```python
from build123d import *

# Parameters (mm, degrees)
F0_W     = 83.5
F0_H     = 70.2625
F0_W_2   = 8
F0_H_2   = 3.175
F0_W_3   = 77.5
F0_H_3   = 24
F0_R     = 1
F0_W_4   = 6
F0_W_5   = 17
F0_H_4   = 31
F0_W_6   = 10
F0_H_5   = 10
F0_R_2   = 1.2
F1_DEPTH = 3.175


# Not quite as in the source:
# - a length typed as a fraction of an inch, garbled in the dataset ("3 / 203.2 mm" for 3/8 in), is restored
# - a feature names something its author has since deleted; it is built from what else it names


with BuildPart() as f1:
    # F0 (on Top) → F1 (new body)
    with BuildSketch(Plane.XY):
        with Locations((2.5199788651, 27.2772044539)):
            Rectangle(F0_W, F0_H)
        with Locations((-12.4800211349, -3.1790455461)):
            Rectangle(F0_W_2, F0_H_2, mode=Mode.SUBTRACT)
        with BuildLine():
            ThreePointArc((-0.9800211349, -4.6790455461), (-2.0406813067, -2.1183853743), (0.5199788651, -3.1790455461))
            ThreePointArc((0.5199788651, -3.1790455461), (0.0806390368, -4.2397057179), (-0.9800211349, -4.6790455461))
        make_face(mode=Mode.SUBTRACT)
        with Locations((10.5199788651, -3.1790455461)):
            Rectangle(F0_W_2, F0_H_2, mode=Mode.SUBTRACT)
        with Locations((2.5199788651, 13.4084544539)):
            Rectangle(F0_W_3, F0_H_3, mode=Mode.SUBTRACT)
        Polygon((-36.2300211349, 34.4084544539), (-36.230021135, 44.4084544539), (-36.230021135, 54.4084544539), (-26.230021135, 54.4084544539), (-26.230021135, 44.4084544539), (-26.2300211349, 34.4084544539), align=None, mode=Mode.SUBTRACT)
        with Locations((-14.980021135, 29.4084544539)):
            Circle(F0_R, mode=Mode.SUBTRACT)
        Polygon((-21.230021135, 31.9084544539), (-21.230021135, 55.9084544539), (-8.730021135, 55.9084544539), (-8.730021135, 43.9084544539), (-8.730021135, 31.9084544539), align=None, mode=Mode.SUBTRACT)
        with Locations((-14.980021135, 58.4084544539)):
            Circle(F0_R, mode=Mode.SUBTRACT)
        with Locations((21.2699788651, 35.3209544539)):
            Rectangle(F0_W_4, F0_H_2, mode=Mode.SUBTRACT)
        with Locations((2.7699788651, 43.9084544539)):
            Rectangle(F0_W_5, F0_H_4, mode=Mode.SUBTRACT)
        with BuildLine():
            ThreePointArc((29.7699788651, 33.8209544539), (28.7093186933, 36.3816146257), (31.2699788651, 35.3209544539))
            ThreePointArc((31.2699788651, 35.3209544539), (30.8306390368, 34.2602942821), (29.7699788651, 33.8209544539))
        make_face(mode=Mode.SUBTRACT)
        with Locations((38.2699788651, 35.3209544539)):
            Rectangle(F0_W_4, F0_H_2, mode=Mode.SUBTRACT)
        Polygon((14.2699788651, 54.4084544539), (24.2699788651, 54.4084544539), (34.2699788651, 54.4084544539), (34.2699788651, 44.4084544539), (24.2699788651, 44.4084544539), (14.2699788651, 44.4084544539), align=None, mode=Mode.SUBTRACT)
        with Locations((-31.2300211349, 39.4084544539)):
            Rectangle(F0_W_6, F0_H_5)
        with Locations((-31.230021135, 39.4084544539)):
            Circle(F0_R_2, mode=Mode.SUBTRACT)
        with Locations((19.2699788651, 49.4084544539)):
            Rectangle(F0_W_6, F0_H_5)
        with Locations((19.2699788651, 49.4084544539)):
            Circle(F0_R_2, mode=Mode.SUBTRACT)
    extrude(amount=F1_DEPTH)


solid = f1.part
```
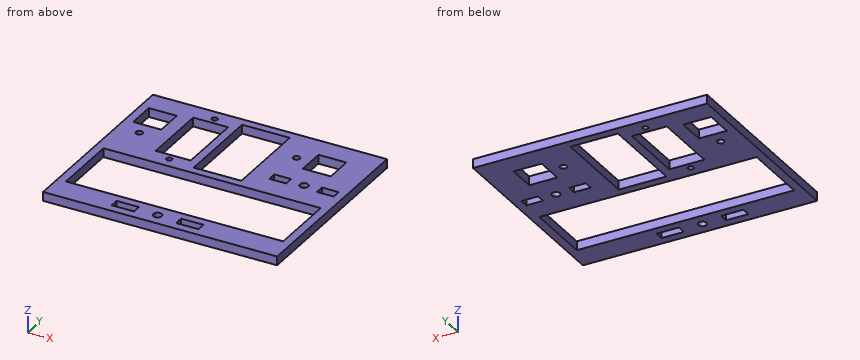
The listing builds one solid part. Answer for the finished solid, in the listing's coordinates (mm). Give positions to 0.01 mm unless a question says otherwise; leave off trailing zeros. Write each loop counter-clockwise with the first axis right and the second up, starting at its lowest first coordinate (ties: lowest second). Pieces come first, ordered by that corner, then holes. Notation, with made-up numbers: (44, 49) -> (69, 49) arc R21 cw to (69, 56) -> close; hole circle Ø2 at (40.5, 34). An arc over 180 degrees is marked (long way). Write item = value, one per line. Start each with the question number.
1) The part is cut by section C-C, the plane x = -4. Determine the outline of the cut face in (y, z) (3 decimals).
2) The part is cut by section B-B, the plane y = 42. Determine the outline of the cut face in (x, z) (3 decimals).
3) The part is cut by section A-A, the plane y = 8.5. Determine the outline of the cut face in (x, z) (3 decimals), and give its area (4 significant figures).
4) Straight lines are drawn through the part: line 1 along X through (y, z) = (33.5, 2.1); line 2 along Y through (x, z) = (25.5, 0.6); line 3 along X through (y, z) = (23, 1.65). For each, find the intervals that lie inside material, in ascending order.
5) The part is cut by section D-D, the plane x = 16. Determine the outline of the cut face in (y, z) (3 decimals), and give its area (3 significant figures).
Solutions:
q1.outline = (-7.854, 0) -> (1.408, 0) -> (1.408, 3.175) -> (-7.854, 3.175) -> close; (25.408, 0) -> (28.408, 0) -> (28.408, 3.175) -> (25.408, 3.175) -> close; (59.408, 0) -> (62.408, 0) -> (62.408, 3.175) -> (59.408, 3.175) -> close
q2.outline = (-39.23, 0) -> (-21.23, 0) -> (-21.23, 3.175) -> (-39.23, 3.175) -> close; (-8.73, 0) -> (-5.73, 0) -> (-5.73, 3.175) -> (-8.73, 3.175) -> close; (11.27, 0) -> (44.27, 0) -> (44.27, 3.175) -> (11.27, 3.175) -> close
q3.outline = (-39.23, 0) -> (-36.23, 0) -> (-36.23, 3.175) -> (-39.23, 3.175) -> close; (41.27, 0) -> (44.27, 0) -> (44.27, 3.175) -> (41.27, 3.175) -> close
q3.area = 19.05 mm²
q4.line_1 = -39.23 to -21.23, -8.73 to -5.73, 11.27 to 44.27
q4.line_2 = -7.85 to 1.41, 25.41 to 44.41, 54.41 to 62.41
q4.line_3 = -39.23 to -36.23, 41.27 to 44.27
q5.outline = (-7.854, 0) -> (1.408, 0) -> (1.408, 3.175) -> (-7.854, 3.175) -> close; (25.408, 0) -> (62.408, 0) -> (62.408, 3.175) -> (25.408, 3.175) -> close
q5.area = 147 mm²
